CAD build for the part. Positions are in the model's coordinates, mm. Give positions to 0.01 mm unless a question says otherwise; leave off trailing zeros. Write each loop counter-clockwise with the first axis right and the second up, starting at its lowest first coordinate (ties: lowest second). Pieces come first, ordered by that corner, then holes. Notation, with made-up numbers: (13.25, 84) - (71.25, 84) arc R31 cw to (71.25, 110) - close; hole circle Ø2 at (89, 63). An arc over 180 degrees is marked (long way). Write item = value, one per line. Start each with the question number.
```python
from build123d import *

# Parameters (mm, degrees)
SALIENTE_EXTRUIR1_DEPTH = 5
CORTAR_EXTRUIR1_DEPTH   = 0.5
REDONDEO1_R             = 2
REDONDEO2_R             = 2


with BuildPart() as part:
    # Croquis2 → Saliente-Extruir1 (new body)
    with BuildSketch(Plane.XY):
        with BuildLine():
            ThreePointArc((-61.331528305, 74.17887931), (-92.135043085, -27.842347885), (-9.986497884, -95.730519481))
            ThreePointArc((-9.986497884, -95.730519481), (0, -86.25), (9.986497884, -95.730519481))
            ThreePointArc((9.986497884, -95.730519481), (92.135043085, -27.842347885), (61.331528305, 74.17887931))
            ThreePointArc((61.331528305, 74.17887931), (40.466763827, 78.9231673), (24.253831648, 64.959375))
            ThreePointArc((24.253831648, 64.959375), (0, 48.75), (-24.253831648, 64.959375))
            ThreePointArc((-24.253831648, 64.959375), (-40.466763827, 78.9231673), (-61.331528305, 74.17887931))
        make_face()
    extrude(amount=SALIENTE_EXTRUIR1_DEPTH)

    # Croquis3 → Cortar-Extruir1 (cut)
    # profile 1 of 2: a face of its own
    with BuildSketch(Plane.XY.offset(5)):
        with BuildLine():
            Line((30.060560178, 27.454508154), (-30.060560178, 27.454508154))
            Line((-30.060560178, 27.454508154), (-30.060560178, 4.954508154))
            Line((-30.060560178, 4.954508154), (0, 4.954508154))
            ThreePointArc((0, 4.954508154), (18.623585271, -51.006906249), (-29.81944868, -17.364815175))
            Line((-29.81944868, -17.364815175), (-37.571846699, -17.364815175))
            ThreePointArc((-37.571846699, -17.364815175), (23.983513651, -56.343925991), (0, 12.454508154))
            Line((0, 12.454508154), (-22.560560178, 12.454508154))
            Line((-22.560560178, 12.454508154), (-22.560560178, 19.954508154))
            Line((-22.560560178, 19.954508154), (30.060560178, 19.954508154))
            Line((30.060560178, 19.954508154), (30.060560178, 27.454508154))
        make_face()
    # profile 2 of 2: a face of its own
    with BuildSketch(Plane.XY.offset(5)):
        Polygon((-5, -6.355312768), (5, -6.355312768), (18.083784961, -42.302716508), (11.698718326, -42.302716508), (6.928526472, -29.196722105), (-6.928526472, -29.196722105), (-11.698718326, -42.302716508), (-18.083784961, -42.302716508), align=None)
        Polygon((-4.744705067, -23.196722105), (4.744705067, -23.196722105), (0.434784536, -11.355312768), (-0.434784536, -11.355312768), align=None, mode=Mode.SUBTRACT)
    extrude(amount=-CORTAR_EXTRUIR1_DEPTH, mode=Mode.SUBTRACT)

    # Redondeo1
    redondeo1_edges = [part.edges().sort_by_distance(p)[0] for p in [
        (-9.986497884, -95.730519481, 2.5),
    ]]
    fillet(redondeo1_edges, radius=REDONDEO1_R)

    # Redondeo2
    redondeo2_edges = [part.edges().sort_by_distance(p)[0] for p in [
        (9.986497884, -95.730519481, 2.5),
    ]]
    fillet(redondeo2_edges, radius=REDONDEO2_R)


solid = part.part
```
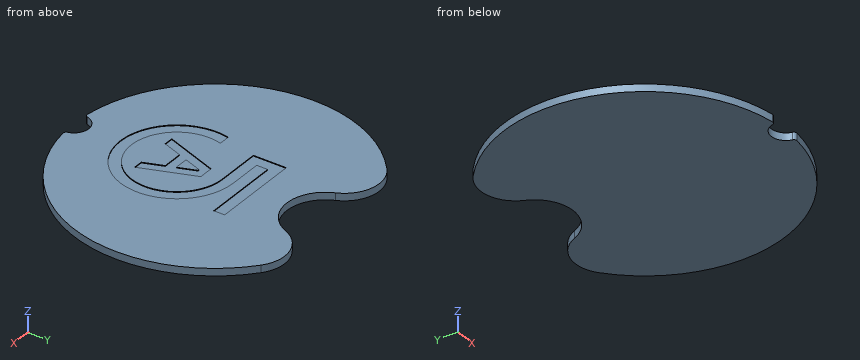
1. Cut at D-D (x = 67). Give the cut face in (y, z), then the cut area to 3 significant figures.
2. Wall check: line 1 along X through (y, z) = (70, 0.4); line 2 along X through (y, z) = (-40.5, 3.9); line 3 along X through (y, z) = (44, 2.9). Give the ranges that are in metal, low to high.
3. Pin check, flat tips, straight feed: pin 1 Ø1.5 at (x, z) = (-67, 1) entering from -Y; pin 2 Ø3 at (y, z) = (-34.5, 2) entering from -X; pin 3 Ø0.6 at (y, z) = (14.5, 4.5) entering from -X. Stop position of each tip, or through.
4. Cut at C-C (y = 24.5). Give the cut face in (x, z), then the cut area to 3 significant figures.
5. Cut at B-B (x = -83.5). Give the cut face in (y, z), then the cut area to 3 significant figures.
6. Cut at A-A (y = -61). Give the cut face in (x, z).
Output:
q1.outline = (-69.1, 0) - (69.1, 0) - (69.1, 5) - (-69.1, 5) - close
q1.area = 691 mm2
q2.line_1 = -66.06 to -27.1, 27.1 to 66.06
q2.line_2 = -87.31 to 87.31
q2.line_3 = -85.6 to 85.6
q3.pin_1 = -69.82
q3.pin_2 = -90.42
q3.pin_3 = -95.2
q4.outline = (-93.08, 0) - (93.08, 0) - (93.08, 5) - (30.06, 5) - (30.06, 4.5) - (-30.06, 4.5) - (-30.06, 5) - (-93.08, 5) - close
q4.area = 901 mm2
q5.outline = (-47.87, 0) - (47.87, 0) - (47.87, 5) - (-47.87, 5) - close
q5.area = 479 mm2
q6.outline = (-74.45, 0) - (74.45, 0) - (74.45, 5) - (16.5, 5) - (16.5, 4.5) - (-16.5, 4.5) - (-16.5, 5) - (-74.45, 5) - close
